```python
from build123d import *

# Parameters (mm, degrees)
SKETCH_2_R               = 1.5
CUT_EXTRUDE_1_DEPTH      = 10
PATTERN_CIRCULAR_1_COUNT = 12


with BuildPart() as part:
    # 草图1 → 旋转1 (revolve)
    with BuildSketch(Plane.XY, mode=Mode.PRIVATE) as revolve_1_sk:
        Polygon((-53, 0), (-59, 0), (-59, 3), (-51.2, 3), (-51.2, 0), align=None)
    revolve(revolve_1_sk.sketch.rotate(Axis((0, 0, 0), (0, 1, 0)), 270), axis=Axis((0, 0, 0), (0, 1, 0)))

    # 草图2 → 切除-拉伸1 (cut)
    with BuildSketch(Plane.XZ):
        with Locations(Location((0, 56, 0), (0, 0, 270))):
            Circle(SKETCH_2_R)
    cut_extrude_1 = extrude(amount=-CUT_EXTRUDE_1_DEPTH, mode=Mode.SUBTRACT)

    # 阵列(圆周)1: 切除-拉伸1 ×12 about axis
    pattern_circular_1_axis = Axis((0, 0, 0), (0, 1, 0))
    for i in range(1, PATTERN_CIRCULAR_1_COUNT):
        add(cut_extrude_1.rotate(pattern_circular_1_axis, i * 360 / PATTERN_CIRCULAR_1_COUNT), mode=Mode.SUBTRACT)

    # 圆角1: read off the stored shape, not the designer's step
    # 圆角1: loft between two sections, ruled curve by curve
    fillet_1_from = [
        Edge.make_three_point_arc((28, 2, 46.997422612), (29.5, 2, 48.497422612), (28, 2, 49.997422612)),
        Edge.make_three_point_arc((28, 2, 49.997422612), (26.5, 2, 48.497422612), (28, 2, 46.997422612)),
    ]
    fillet_1_to = [
        Edge.make_three_point_arc((28, 0, 44.997422612), (31.5, 0, 48.497422612), (28, 0, 51.997422612)),
        Edge.make_three_point_arc((28, 0, 51.997422612), (24.5, 0, 48.497422612), (28, 0, 44.997422612)),
    ]
    fillet_1 = Solid(Shell([*[Face.make_surface_from_curves(fillet_1_from[k], fillet_1_to[k]) for k in range(2)], Face(Wire(fillet_1_from)), Face(Wire(fillet_1_to))]))
    add(fillet_1, mode=Mode.SUBTRACT)

    # Fillet 1 2: loft between two sections, ruled curve by curve
    fillet_1_2_from = [
        Edge.make_three_point_arc((48.497422612, 2, 26.5), (49.997422612, 2, 28), (48.497422612, 2, 29.5)),
        Edge.make_three_point_arc((48.497422612, 2, 29.5), (46.997422612, 2, 28), (48.497422612, 2, 26.5)),
    ]
    fillet_1_2_to = [
        Edge.make_three_point_arc((48.497422612, 0, 24.5), (51.997422612, 0, 28), (48.497422612, 0, 31.5)),
        Edge.make_three_point_arc((48.497422612, 0, 31.5), (44.997422612, 0, 28), (48.497422612, 0, 24.5)),
    ]
    fillet_1_2 = Solid(Shell([*[Face.make_surface_from_curves(fillet_1_2_from[k], fillet_1_2_to[k]) for k in range(2)], Face(Wire(fillet_1_2_from)), Face(Wire(fillet_1_2_to))]))
    add(fillet_1_2, mode=Mode.SUBTRACT)

    # Fillet 1 3: loft between two sections, ruled curve by curve
    fillet_1_3_from = [
        Edge.make_three_point_arc((56, 2, -1.5), (57.5, 2, 0), (56, 2, 1.5)),
        Edge.make_three_point_arc((56, 2, 1.5), (54.5, 2, 0), (56, 2, -1.5)),
    ]
    fillet_1_3_to = [
        Edge.make_three_point_arc((56, 0, -3.5), (59.5, 0, 0), (56, 0, 3.5)),
        Edge.make_three_point_arc((56, 0, 3.5), (52.5, 0, 0), (56, 0, -3.5)),
    ]
    fillet_1_3 = Solid(Shell([*[Face.make_surface_from_curves(fillet_1_3_from[k], fillet_1_3_to[k]) for k in range(2)], Face(Wire(fillet_1_3_from)), Face(Wire(fillet_1_3_to))]))
    add(fillet_1_3, mode=Mode.SUBTRACT)

    # Fillet 1 4: loft between two sections, ruled curve by curve
    fillet_1_4_from = [
        Edge.make_three_point_arc((48.497422612, 2, -29.5), (49.997422612, 2, -28), (48.497422612, 2, -26.5)),
        Edge.make_three_point_arc((48.497422612, 2, -26.5), (46.997422612, 2, -28), (48.497422612, 2, -29.5)),
    ]
    fillet_1_4_to = [
        Edge.make_three_point_arc((48.497422612, 0, -31.5), (51.997422612, 0, -28), (48.497422612, 0, -24.5)),
        Edge.make_three_point_arc((48.497422612, 0, -24.5), (44.997422612, 0, -28), (48.497422612, 0, -31.5)),
    ]
    fillet_1_4 = Solid(Shell([*[Face.make_surface_from_curves(fillet_1_4_from[k], fillet_1_4_to[k]) for k in range(2)], Face(Wire(fillet_1_4_from)), Face(Wire(fillet_1_4_to))]))
    add(fillet_1_4, mode=Mode.SUBTRACT)

    # Fillet 1 5: loft between two sections, ruled curve by curve
    fillet_1_5_from = [
        Edge.make_three_point_arc((28, 2, -49.997422612), (29.5, 2, -48.497422612), (28, 2, -46.997422612)),
        Edge.make_three_point_arc((28, 2, -46.997422612), (26.5, 2, -48.497422612), (28, 2, -49.997422612)),
    ]
    fillet_1_5_to = [
        Edge.make_three_point_arc((28, 0, -51.997422612), (31.5, 0, -48.497422612), (28, 0, -44.997422612)),
        Edge.make_three_point_arc((28, 0, -44.997422612), (24.5, 0, -48.497422612), (28, 0, -51.997422612)),
    ]
    fillet_1_5 = Solid(Shell([*[Face.make_surface_from_curves(fillet_1_5_from[k], fillet_1_5_to[k]) for k in range(2)], Face(Wire(fillet_1_5_from)), Face(Wire(fillet_1_5_to))]))
    add(fillet_1_5, mode=Mode.SUBTRACT)

    # Fillet 1 6: loft between two sections, ruled curve by curve
    fillet_1_6_from = [
        Edge.make_three_point_arc((0, 2, -57.5), (1.5, 2, -56), (0, 2, -54.5)),
        Edge.make_three_point_arc((0, 2, -54.5), (-1.5, 2, -56), (0, 2, -57.5)),
    ]
    fillet_1_6_to = [
        Edge.make_three_point_arc((0, 0, -59.5), (3.5, 0, -56), (0, 0, -52.5)),
        Edge.make_three_point_arc((0, 0, -52.5), (-3.5, 0, -56), (0, 0, -59.5)),
    ]
    fillet_1_6 = Solid(Shell([*[Face.make_surface_from_curves(fillet_1_6_from[k], fillet_1_6_to[k]) for k in range(2)], Face(Wire(fillet_1_6_from)), Face(Wire(fillet_1_6_to))]))
    add(fillet_1_6, mode=Mode.SUBTRACT)

    # Fillet 1 7: loft between two sections, ruled curve by curve
    fillet_1_7_from = [
        Edge.make_three_point_arc((-28, 2, -49.997422612), (-26.5, 2, -48.497422612), (-28, 2, -46.997422612)),
        Edge.make_three_point_arc((-28, 2, -46.997422612), (-29.5, 2, -48.497422612), (-28, 2, -49.997422612)),
    ]
    fillet_1_7_to = [
        Edge.make_three_point_arc((-28, 0, -51.997422612), (-24.5, 0, -48.497422612), (-28, 0, -44.997422612)),
        Edge.make_three_point_arc((-28, 0, -44.997422612), (-31.5, 0, -48.497422612), (-28, 0, -51.997422612)),
    ]
    fillet_1_7 = Solid(Shell([*[Face.make_surface_from_curves(fillet_1_7_from[k], fillet_1_7_to[k]) for k in range(2)], Face(Wire(fillet_1_7_from)), Face(Wire(fillet_1_7_to))]))
    add(fillet_1_7, mode=Mode.SUBTRACT)

    # Fillet 1 8: loft between two sections, ruled curve by curve
    fillet_1_8_from = [
        Edge.make_three_point_arc((-48.497422612, 2, -29.5), (-46.997422612, 2, -28), (-48.497422612, 2, -26.5)),
        Edge.make_three_point_arc((-48.497422612, 2, -26.5), (-49.997422612, 2, -28), (-48.497422612, 2, -29.5)),
    ]
    fillet_1_8_to = [
        Edge.make_three_point_arc((-48.497422612, 0, -31.5), (-44.997422612, 0, -28), (-48.497422612, 0, -24.5)),
        Edge.make_three_point_arc((-48.497422612, 0, -24.5), (-51.997422612, 0, -28), (-48.497422612, 0, -31.5)),
    ]
    fillet_1_8 = Solid(Shell([*[Face.make_surface_from_curves(fillet_1_8_from[k], fillet_1_8_to[k]) for k in range(2)], Face(Wire(fillet_1_8_from)), Face(Wire(fillet_1_8_to))]))
    add(fillet_1_8, mode=Mode.SUBTRACT)

    # Fillet 1 9: loft between two sections, ruled curve by curve
    fillet_1_9_from = [
        Edge.make_three_point_arc((-56, 2, -1.5), (-54.5, 2, 0), (-56, 2, 1.5)),
        Edge.make_three_point_arc((-56, 2, 1.5), (-57.5, 2, 0), (-56, 2, -1.5)),
    ]
    fillet_1_9_to = [
        Edge.make_three_point_arc((-56, 0, -3.5), (-52.5, 0, 0), (-56, 0, 3.5)),
        Edge.make_three_point_arc((-56, 0, 3.5), (-59.5, 0, 0), (-56, 0, -3.5)),
    ]
    fillet_1_9 = Solid(Shell([*[Face.make_surface_from_curves(fillet_1_9_from[k], fillet_1_9_to[k]) for k in range(2)], Face(Wire(fillet_1_9_from)), Face(Wire(fillet_1_9_to))]))
    add(fillet_1_9, mode=Mode.SUBTRACT)

    # Fillet 1 10: loft between two sections, ruled curve by curve
    fillet_1_10_from = [
        Edge.make_three_point_arc((-48.497422612, 2, 26.5), (-46.997422612, 2, 28), (-48.497422612, 2, 29.5)),
        Edge.make_three_point_arc((-48.497422612, 2, 29.5), (-49.997422612, 2, 28), (-48.497422612, 2, 26.5)),
    ]
    fillet_1_10_to = [
        Edge.make_three_point_arc((-48.497422612, 0, 24.5), (-44.997422612, 0, 28), (-48.497422612, 0, 31.5)),
        Edge.make_three_point_arc((-48.497422612, 0, 31.5), (-51.997422612, 0, 28), (-48.497422612, 0, 24.5)),
    ]
    fillet_1_10 = Solid(Shell([*[Face.make_surface_from_curves(fillet_1_10_from[k], fillet_1_10_to[k]) for k in range(2)], Face(Wire(fillet_1_10_from)), Face(Wire(fillet_1_10_to))]))
    add(fillet_1_10, mode=Mode.SUBTRACT)

    # Fillet 1 11: loft between two sections, ruled curve by curve
    fillet_1_11_from = [
        Edge.make_three_point_arc((-28, 2, 46.997422612), (-26.5, 2, 48.497422612), (-28, 2, 49.997422612)),
        Edge.make_three_point_arc((-28, 2, 49.997422612), (-29.5, 2, 48.497422612), (-28, 2, 46.997422612)),
    ]
    fillet_1_11_to = [
        Edge.make_three_point_arc((-28, 0, 44.997422612), (-24.5, 0, 48.497422612), (-28, 0, 51.997422612)),
        Edge.make_three_point_arc((-28, 0, 51.997422612), (-31.5, 0, 48.497422612), (-28, 0, 44.997422612)),
    ]
    fillet_1_11 = Solid(Shell([*[Face.make_surface_from_curves(fillet_1_11_from[k], fillet_1_11_to[k]) for k in range(2)], Face(Wire(fillet_1_11_from)), Face(Wire(fillet_1_11_to))]))
    add(fillet_1_11, mode=Mode.SUBTRACT)

    # Fillet 1 12: loft between two sections, ruled curve by curve
    fillet_1_12_from = [
        Edge.make_three_point_arc((0, 2, 54.5), (1.5, 2, 56), (0, 2, 57.5)),
        Edge.make_three_point_arc((0, 2, 57.5), (-1.5, 2, 56), (0, 2, 54.5)),
    ]
    fillet_1_12_to = [
        Edge.make_three_point_arc((0, 0, 52.5), (3.5, 0, 56), (0, 0, 59.5)),
        Edge.make_three_point_arc((0, 0, 59.5), (-3.5, 0, 56), (0, 0, 52.5)),
    ]
    fillet_1_12 = Solid(Shell([*[Face.make_surface_from_curves(fillet_1_12_from[k], fillet_1_12_to[k]) for k in range(2)], Face(Wire(fillet_1_12_from)), Face(Wire(fillet_1_12_to))]))
    add(fillet_1_12, mode=Mode.SUBTRACT)


solid = part.part
```
Read the model definition and answer for the solid it produces. Units are mm, in the model's axes. Round coordinates to 2 decimals unless told otherwise and drop trailing zeros. Loops run counter-clockwise (first coordinate to the right, second up) from the corner with the lowest first, then second, coordinate; pieces in that order, holes last. Notation, with made-up numbers: (24, 24) -> (50, 24) arc R23 ccw to (50, 41) -> close; hole circle Ø6 at (84, 14). An arc over 180 degrees is marked (long way). One line per item, written item: value.
1) A cutting plane is placed at A-A (z = -33). Determine the outline of the cut face in (x, y), and give its area (3 significant figures).
Answer list:
outline: (-48.91, 0) -> (-39.15, 0) -> (-39.15, 3) -> (-48.91, 3) -> close; (39.15, 0) -> (48.91, 0) -> (48.91, 3) -> (39.15, 3) -> close
area: 58.6 mm²
2) Flat-ended cylindrical pins translate along their axes: P1, Ø3.5, axis at x = 48.5, z = -28, coming from the -Y side; P2, Ø5, axis at x = -48.5, z = -28, coming from the -Y side; P3, Ø1.5, axis at y = 2, z = 3.5, coming from the -X side. Find the tip coordinate at first contact, or state that the pin passes through.
Answer list:
P1: stops at y = 1.75
P2: stops at y = 1
P3: stops at x = -58.94
3) Consider L1, parallel to X at y = 0.95, z = 29; L2, parallel to Z at x = 27, y = 0.45; L3, parallel to X at y = 1.1, z = 29. Determine where each line is inside the solid, lowest interval first. Write a range as [from, to].
Answer list:
L1: x = [-51.38, -50.84], [-46.15, -42.2], [42.2, 46.15], [50.84, 51.38]
L2: z = [-52.46, -51.38], [-45.62, -43.5], [43.5, 45.62], [51.38, 52.46]
L3: x = [-51.38, -50.68], [-46.32, -42.2], [42.2, 46.32], [50.68, 51.38]
4) A cutting plane is placed at B-B (x = 12). Determine the outline of the cut face in (y, z), and give its area (3 significant figures).
Answer list:
outline: (0, -57.77) -> (3, -57.77) -> (3, -49.77) -> (0, -49.77) -> close; (0, 49.77) -> (3, 49.77) -> (3, 57.77) -> (0, 57.77) -> close
area: 48.0 mm²
5) A cutting plane is placed at C-C (z = 0). Give the number of separate pieces and of enclosed holes in the cut face, and give its area (4 significant figures).
Answer list:
separate pieces: 4
enclosed holes: 0
area: 21.05 mm²
6) The mould has two halves that part along X. Classify faces 1 (the face through (-47.484, 2.493, -26.894)), 2 (the face through (52, 0, 0)), 3 (the face through (47.484, 2.493, 26.894)), 4 (the face through (-17.722, 1.521, -56.275)): pulls with the +X half, pulls with the -X half, needs draft (parallel to the pull), parting line crosses it, or undercut.
Answer list:
face 1: undercut
face 2: needs draft
face 3: undercut
face 4: parting line crosses it
